Work out the finished part from the listing and answer in its coordinate system (mm). Coordinates: 2 decimals unless noted, no trailing zeros. Order: outer loops, then holes, each group sorted by start corner. A loop starts at its lowest first (then second) coordinate and runs counter-clockwise, first axis right, second up.
```python
from build123d import *

# Parameters (mm, degrees)
BOX021_W               = 10
BOX021_H               = 100
BOX021_DEPTH           = 10
BOX021_PLACEMENT_ANGLE = 310
BOX022_W               = 16
BOX022_H               = 102
BOX022_DEPTH           = 3
BOX022_PLACEMENT_ANGLE = 310
BOX023_W               = 3
BOX023_H               = 102
BOX023_DEPTH           = 2
BOX009_W               = 14
BOX009_H               = 96
BOX009_DEPTH           = 5
BOX008_W               = 15
BOX008_H               = 96
BOX008_DEPTH           = 10
FILLET_R               = 1
FILLET_PLACEMENT_ANGLE = 311


with BuildPart() as cube021:
    # Box021 → Box021 (new body)
    with BuildSketch(Plane.XY):
        with Locations((5, 50)):
            Rectangle(BOX021_W, BOX021_H)
    extrude(amount=BOX021_DEPTH)


with BuildPart() as cube021_1:
    # Box021 placement: moved
    add(cube021.part.moved(Location((25, 1, -35))).rotate(Axis((25, 1, -35), (0, 1, 0)), BOX021_PLACEMENT_ANGLE))


with BuildPart() as cube022:
    # Box022 → Box022 (new body)
    with BuildSketch(Plane.XY):
        with Locations((8, 51)):
            Rectangle(BOX022_W, BOX022_H)
    extrude(amount=BOX022_DEPTH)


with BuildPart() as cube022_1:
    # Box022 placement: moved
    add(cube022.part.moved(Location((15.5, 0, -22))).rotate(Axis((15.5, 0, -22), (0, 1, 0)), BOX022_PLACEMENT_ANGLE))


with BuildPart() as fusion001:
    # Box023 → Box023 (new body)
    with BuildSketch(Plane(origin=(25.98, 0, -9.95), x_dir=(0, 0, 1), z_dir=(-1, 0, 0))):
        with Locations((1.5, 51)):
            Rectangle(BOX023_W, BOX023_H)
    extrude(amount=BOX023_DEPTH)

    # Fusion001: union Cube022
    add(cube022_1.part)


with BuildPart() as cube009:
    # Box009 → Box009 (new body)
    with BuildSketch(Plane(origin=(14, 2, -21), x_dir=(1, 0, 0), z_dir=(0, 0, 1))):
        with Locations((7, 48)):
            Rectangle(BOX009_W, BOX009_H)
    extrude(amount=BOX009_DEPTH)


with BuildPart() as cut013:
    # Box008 → Box008 (new body)
    with BuildSketch(Plane(origin=(13, 2, -21), x_dir=(1, 0, 0), z_dir=(0, 0, 1))):
        with Locations((7.5, 48)):
            Rectangle(BOX008_W, BOX008_H)
    extrude(amount=BOX008_DEPTH)

    # Cut002: cut Cube009
    add(cube009.part, mode=Mode.SUBTRACT)

    # Fillet
    fillet_edges = [cut013.edges().sort_by_distance(p)[0] for p in [
        (14, 50, -16),
    ]]
    fillet(fillet_edges, radius=FILLET_R)


with BuildPart() as cut013_1:
    # Fillet placement: moved
    add(cut013.part.moved(Location((-1.63, 0, -23.03))).rotate(Axis((-1.63, 0, -23.03), (0, 1, 0)), FILLET_PLACEMENT_ANGLE))

    # Cut012: cut Fusion001
    add(fusion001.part, mode=Mode.SUBTRACT)

    # Cut013: cut Cube021
    add(cube021_1.part, mode=Mode.SUBTRACT)


solid = cut013_1.part
```
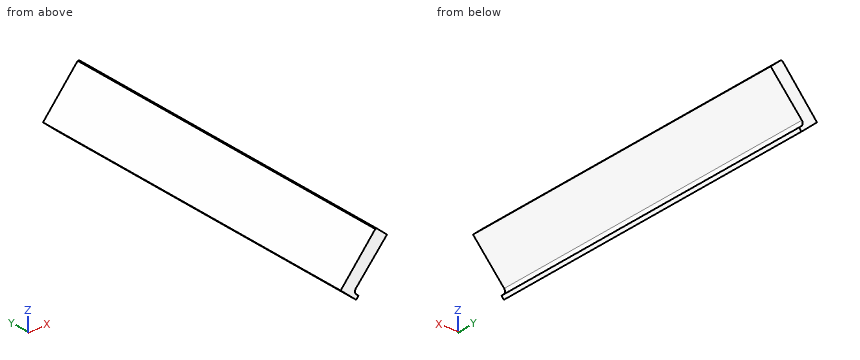
1. Consider probe 1 along X at (y, z) = (82.5, -11.5); probe 2 along Z at (x, y) = (22.75, 72); probe 3 along Z at (x, y) = (22, 82.5). Determine where each line is inside the solid, lowest interval first.
2. The part is cut by section B-B (x = 24.25). Determine the outline of the cut face in (y, z), plus the area to 3 significant figures.
3. The part is cut by section A-A (y = 12.5). Determine the outline of the cut face in (x, z) (3 decimals), plus the area to 3 significant figures.
4. Flat-ended cylindrical pins translate along their axes: pin 1 (3 mm diameter, centred on y = 32, z = -16, fed in from +X); pin 2 (3 mm diameter, centred on x = 17.5, z = -18, fed in from +Y); pin 3 (1 mm diameter, centred on x = 25, y = 60.5, fed in from +Z); pin 4 (2 mm diameter, centred on x = 18.5, y = 65, fed in from -Z). Find the tip coordinate at first contact, or state that the pin passes through.
5. The part is cut by section C-C (z = -11.25). Determine the outline of the cut face in (x, y).
Worked out:
1. probe 1: x = 24.31 to 27.79
1. probe 2: z = -19.37 to -13.36
1. probe 3: z = -20.23 to -14.25
2. outline: (2, -17.65) - (98, -17.65) - (98, -11.57) - (2, -11.57) - close
2. area: 583 mm2
3. outline: (16.133, -21.246) - (20.385, -24.942) - (21.028, -24.176) - (20.385, -23.617) arc R1 cw to (20.286, -22.206) - (28.815, -12.395) - (25.98, -9.931) - (25.98, -9.95) - (25.611, -9.95) - close
3. area: 60.5 mm2
4. pin 1: stops at x = 26.99
4. pin 2: stops at y = 98
4. pin 3: stops at z = -10.08
4. pin 4: stops at z = -24.17
5. outline: (24.52, 2) - (27.5, 2) - (27.5, 98) - (24.52, 98) - close
